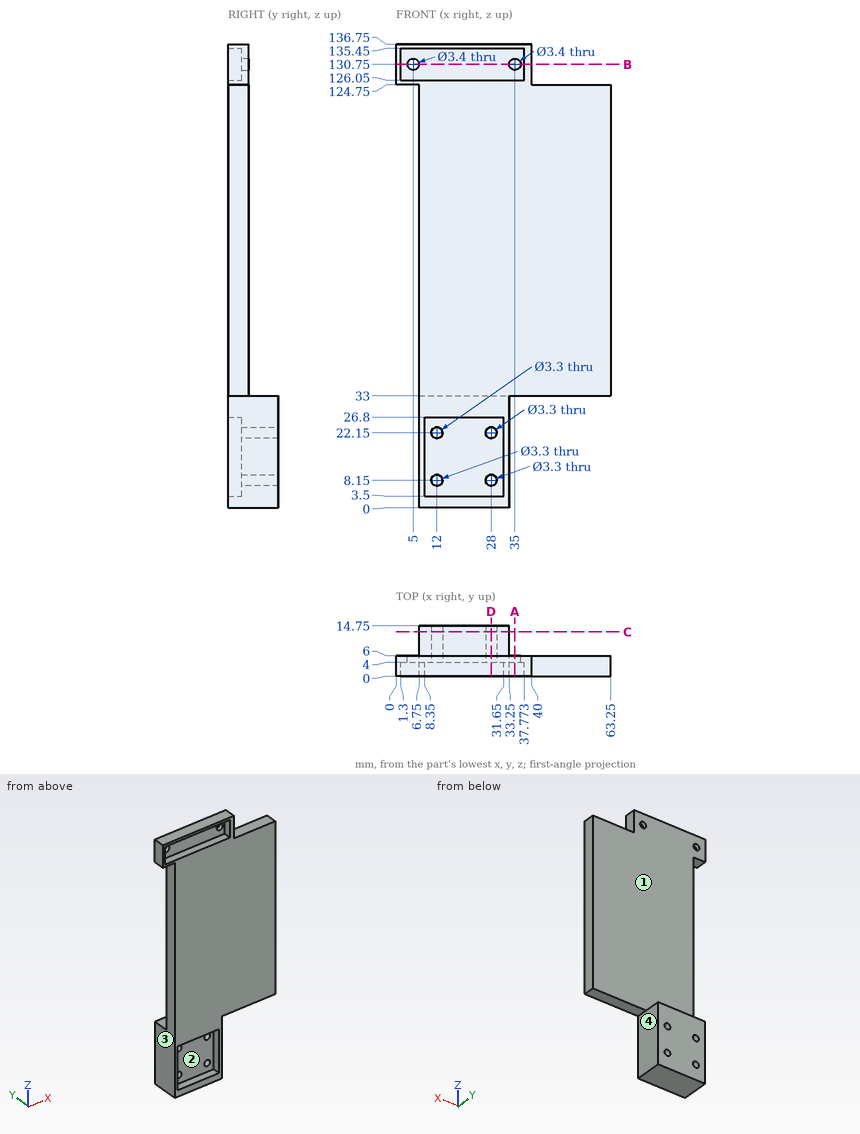
Print and shaded views of the part. All mm, measured from the part's lowest x, y and z. Round coordinates to 2 decimals unless told otherwise and drop trailing zeros. Order: outer loops, then holes, each group sorted by start corner. A loop starts at its lowest first (then second) coordinate and runs counter-clockwise, first axis right, second up. Notation, with made-up numbers: (39.25, 89) - (46.25, 89) arc R32 ccw to (46.25, 121) - close; hole circle Ø9 at (83.25, -1). An arc over 180 degrees is marked (long way). Use a Markdown table: item, result.
1) Saw through at C-C on y = 13. Write the cut outline in (x, z), and give its area (3 significant figures).
Recorded:
| item | result |
|---|---|
| outline | (6.75, 0) - (33.25, 0) - (33.25, 33) - (6.75, 33) - close; hole circle Ø3.3 at (12, 8.15); hole circle Ø3.3 at (12, 22.15); hole circle Ø3.3 at (28, 8.15); hole circle Ø3.3 at (28, 22.15) |
| area | 840 mm² |
2) Wall check: L1, parallel to X at y = 5.55, z = 130.75; L2, parallel to Z at x = 28, y = 9.5; L3, parallel to X at y = 11.5, z = 22.15. Give the ranges that are in metal, low to high.
Recorded:
| item | result |
|---|---|
| L1 | x = 0 to 3.3, 6.7 to 33.3, 36.7 to 40 |
| L2 | z = 0 to 6.5, 9.8 to 20.5, 23.8 to 33 |
| L3 | x = 6.75 to 10.35, 13.65 to 26.35, 29.65 to 33.25 |
3) Pull direction X, two halves, no side cores. Call the marked faces 1, 2, 3 and 4: pulls with the +X half, pulls with the -X half, needs draft (parallel to the pull), parting line crosses it, or undercut.
Recorded:
| item | result |
|---|---|
| face 1 | needs draft |
| face 2 | undercut |
| face 3 | pulls with the -X half |
| face 4 | pulls with the +X half |
4) Saw through at B-B on z = 130.75. Write the cut outline in (x, y).
Recorded:
| item | result |
|---|---|
| outline | (0, 0) - (1.3, 0) - (1.3, 4) - (3.3, 4) - (3.3, 6) - (0, 6) - close; (6.7, 4) - (33.3, 4) - (33.3, 6) - (6.7, 6) - close; (36.7, 4) - (37.77, 4) - (37.77, 0) - (40, 0) - (40, 6) - (36.7, 6) - close |
5) Saw through at A-A on x = 35. Write the cut outline in (y, z).
Recorded:
| item | result |
|---|---|
| outline | (0, 33) - (6, 33) - (6, 129.05) - (4, 129.05) - (4, 126.05) - (0, 126.05) - close; (0, 135.45) - (4, 135.45) - (4, 132.45) - (6, 132.45) - (6, 136.75) - (0, 136.75) - close |
6) Flat gauge pins, fed straight in: pin 1 Ø6.5 at (y, z) = (3, 130.5) entering from +X; pin 2 Ø6 at (y, z) = (1.5, 20.5) entering from +X; pin 3 Ø8 at (x, z) = (19, 65) entering from +Y; pin 4 Ø2.5 at (x, z) = (12, 8.15) entering from -Y. Where does each tip first touch, or does it go through?
Recorded:
| item | result |
|---|---|
| pin 1 | stops at x = 40 |
| pin 2 | stops at x = 33.25 |
| pin 3 | stops at y = 6 |
| pin 4 | passes through |
7) Saw through at D-D on x = 28. Write the cut outline in (y, z).
Recorded:
| item | result |
|---|---|
| outline | (0, 0) - (14.75, 0) - (14.75, 6.5) - (4, 6.5) - (4, 3.5) - (0, 3.5) - close; (0, 26.8) - (4, 26.8) - (4, 23.8) - (14.75, 23.8) - (14.75, 33) - (6, 33) - (6, 136.75) - (0, 136.75) - (0, 135.45) - (4, 135.45) - (4, 126.05) - (0, 126.05) - close; (4, 9.8) - (14.75, 9.8) - (14.75, 20.5) - (4, 20.5) - close |
